```python
from build123d import *

# Parameters (mm, degrees)
SKETCH_W        = 114
SKETCH_H        = 42
PAD_DEPTH       = 39
SKETCH005_W     = 108
SKETCH005_H     = 33
POCKET_DEPTH    = 31
SKETCH007_R     = 13
POCKET001_DEPTH = 39.001
SKETCH006_R     = 1.75
SKETCH006_R_2   = 15
POCKET002_DEPTH = 11.001
POCKET003_DEPTH = 6
POCKET004_DEPTH = 6
SKETCH008_R     = 13
POCKET005_DEPTH = 114.001


with BuildPart() as part:
    # Sketch → Pad (new body)
    with BuildSketch(Plane.XZ):
        with Locations((0, 21)):
            Rectangle(SKETCH_W, SKETCH_H)
    extrude(amount=PAD_DEPTH)

    # Sketch005 → Pocket (cut)
    with BuildSketch(Plane(origin=(0, 0, 42), x_dir=(-1, 0, 0), z_dir=(0, 0, 1))):
        with Locations((0, 19.5)):
            Rectangle(SKETCH005_W, SKETCH005_H)
    extrude(amount=-POCKET_DEPTH, mode=Mode.SUBTRACT)

    # Sketch007 → Pocket001 (cut, through all)
    with BuildSketch(Plane.XZ.offset(39)):
        with Locations((-23, 26)):
            Circle(SKETCH007_R)
        with Locations((8, 26)):
            Circle(SKETCH007_R)
        with Locations((39, 26)):
            Circle(SKETCH007_R)
        with BuildLine():
            ThreePointArc((-42, 33.999986), (-47, 39), (-52, 33.999986))
            Line((-52, 33.999986), (-52, 17.000019))
            ThreePointArc((-52, 17.000019), (-47, 12), (-42, 17.000019))
            Line((-42, 33.999986), (-42, 17.000019))
        make_face()
    extrude(amount=-POCKET001_DEPTH, mode=Mode.SUBTRACT)

    # Sketch006 → Pocket002 (cut, through all)
    with BuildSketch(Plane(origin=(0, 0, 11), x_dir=(-1, 0, 0), z_dir=(0, 0, 1))):
        with Locations((-40, 29)):
            Circle(SKETCH006_R)
        with Locations((40, 29)):
            Circle(SKETCH006_R)
        with Locations((-40, 9)):
            Circle(SKETCH006_R)
        with Locations((40, 9)):
            Circle(SKETCH006_R)
        with Locations((-20, 19.5)):
            Circle(SKETCH006_R_2)
        with Locations((20, 19.5)):
            Circle(SKETCH006_R_2)
    extrude(amount=-POCKET002_DEPTH, mode=Mode.SUBTRACT)

    # Sketch010 → Pocket003 (cut)
    with BuildSketch(Plane(origin=(0, 0, 11), x_dir=(-1, 0, 0), z_dir=(0, 0, 1))):
        Polygon((-42.309401, 13), (-37.690599, 13), (-35.381198, 9), (-37.690599, 5), (-42.309401, 5), (-44.618802, 9), align=None)
    extrude(amount=-POCKET003_DEPTH, mode=Mode.SUBTRACT)

    # Sketch011 → Pocket004 (cut)
    with BuildSketch(Plane(origin=(0, 0, 11), x_dir=(-1, 0, 0), z_dir=(0, 0, 1))):
        Polygon((-42.367136, 33.1), (-37.632864, 33.1), (-35.265728, 29), (-37.632864, 24.9), (-42.367136, 24.9), (-44.734272, 29), align=None)
        Polygon((37.632864, 33.1), (42.367136, 33.1), (44.734272, 29), (42.367136, 24.9), (37.632864, 24.9), (35.265728, 29), align=None)
        Polygon((37.632864, 13.1), (42.367136, 13.1), (44.734272, 9), (42.367136, 4.9), (37.632864, 4.9), (35.265728, 9), align=None)
    extrude(amount=-POCKET004_DEPTH, mode=Mode.SUBTRACT)

    # Sketch008 → Pocket005 (cut, through all)
    with BuildSketch(Plane(origin=(-57, 0, 0), x_dir=(0, 0, -1), z_dir=(-1, 0, 0))):
        with Locations((-25, 19)):
            Circle(SKETCH008_R)
    extrude(amount=-POCKET005_DEPTH, mode=Mode.SUBTRACT)


solid = part.part
```
CAD build for the part. Positions are in the model's coordinates, mm. A direction names the side the tool comes from. Round coordinates to 2 decimals unless told otherwise and drop trailing zeros. Loops run counter-clockwise (first coordinate to the right, second up) from the corner with the lowest first, then second, coordinate; pieces in that order, holes last. Notation, with made-up numbers: M -24,14.5 L -18,14.5 A15 cw -18,40.5 Z; hole C 2.5,-34.5 d2. An arc over 180 degrees is marked long. Use a Markdown table: item, result. Add a question column.
(1) Cut at B-B (y = -16). Give the cut face in (x, z).
(2) Flat gauge pins, fed straight in: pin 1 (4 mm diameter, centred on x = -39, z = 8.5, fed in from +Y); pin 2 (12 mm diameter, centred on x = -6.5, y = -18, fed in from +Z); pin 3 (1.5 mm diameter, centred on x = -7, y = -15.5, fed in from -Z); pin 4 (5.5 mm diameter, centred on x = 40, y = -9, fed in from +Z). Where does each tip first touch, or does it go through?
(3) Pull direction Z, two halves, no side cores. Call faces 1 (the face through (-47, -38, 12)), 2 (the face through (36.466, -31.079, 8.042)), 3 (the face through (42, -29, 5)): +Z half, -Z half, draft (parallel to the pull), parting line (faces both ways), or undercut.
(4) Drill centre lines: line 1 (Z direction, x = 55.4, y = -19); line 2 (Y direction, x = -40, z = 2); line 3 (Y direction, x = 52.5, z = 16.5). Where is each one in solid material? Low to high.
(5) Cut at C-C (z = 28.5). State how many separate pieces and enclosed holes the cut face has, and give its area (3 significant figures).
(6) Which spindle directions (+Z, -Z, +X, -X, +Y, -Y) get a long thin tool onto all of the face, cutting with end or side? Do faces 4 (the face through (-36.43, -11.02, 8.04)), 5 (the face through (-52, -2, 26)), 6 (the face through (-16.748, -4.857, 5.577)). Say none if no direction does.
(7) Cut at A-A (x = 8). Give the cut face in (y, z).
(8) Cut at D-D (x = 48). Give the cut face in (y, z).
Geometry says:
| question | item | result |
|---|---|---|
| 1 | outline | M -57,0 L -34.59,0 L -34.59,11 L -54,11 L -54,12.35 L -57,12.35 Z; M -57,37.65 L -54,37.65 L -54,42 L -57,42 Z; M -5.41,0 L 5.41,0 L 5.41,11 L -5.41,11 Z; M 34.59,0 L 57,0 L 57,12.35 L 54,12.35 L 54,11 L 34.59,11 Z; M 54,37.65 L 57,37.65 L 57,42 L 54,42 Z |
| 2 | pin 1 | stops at y = 0 |
| 2 | pin 2 | stops at z = 11 |
| 2 | pin 3 | passes through |
| 2 | pin 4 | stops at z = 5 |
| 3 | face 1 | undercut |
| 3 | face 2 | draft |
| 3 | face 3 | +Z half |
| 4 | line 1 | z = 0 to 12, 38 to 42 |
| 4 | line 2 | y = -39 to -30.75, -27.25 to -10.75, -7.25 to 0 |
| 4 | line 3 | y = -39 to -36, -3 to 0 |
| 5 | separate pieces | 10 |
| 5 | enclosed holes | 0 |
| 5 | area | 212 mm² |
| 6 | face 4 | +Z |
| 6 | face 5 | +Y, -Y |
| 6 | face 6 | +Z, -Z |
| 7 | outline | M -39,0 L -28.5,0 L -28.5,11 L -36,11 L -36,13 L -39,13 Z; M -39,39 L -36,39 L -36,42 L -39,42 Z; M -10.5,0 L 0,0 L 0,13 L -3,13 L -3,11 L -10.5,11 Z; M -3,39 L 0,39 L 0,42 L -3,42 Z |
| 8 | outline | M -39,0 L 0,0 L 0,16.62 L -3,16.62 L -3,11 L -36,11 L -36,16.62 L -39,16.62 Z; M -39,35.38 L -36,35.38 L -36,42 L -39,42 Z; M -3,35.38 L 0,35.38 L 0,42 L -3,42 Z |
